```python
from build123d import *

# Parameters (mm, degrees)
F0_W     = 127
F0_H     = 63.5
F0_R     = 19.05
F1_DEPTH = 25.4
F2_W     = 6.35
F2_H     = 63.5
F2_W_2   = 12.7
F3_DEPTH = 2.54
F5_DEPTH = 66.04
F6_R     = 4.7625
F7_DEPTH = 12.7


with BuildPart() as f1:
    # F0 (on Front) → F1 (new body)
    with BuildSketch(Plane.XZ):
        with Locations((1.798787, 0)):
            Rectangle(F0_W, F0_H)
        Circle(F0_R, mode=Mode.SUBTRACT)
    extrude(amount=F1_DEPTH)

    # F2 (on face) → F3 (cut)
    with BuildSketch(Plane.XZ.offset(25.4)):
        with Locations((-55.986213, 0)):
            Rectangle(F2_W, F2_H)
        Rectangle(F2_W_2, F2_H)
    extrude(amount=-F3_DEPTH, mode=Mode.SUBTRACT)

    # F4 (on face) → F5 (cut)
    with BuildSketch(Plane(origin=(0, 0, -31.75), x_dir=(1, 0, 0), z_dir=(0, 0, -1))):
        Polygon((44.45, 25.4), (31.75, 25.4), (28.817061, 20.32), (47.382939, 20.32), align=None)
    extrude(amount=-F5_DEPTH, mode=Mode.SUBTRACT)

    # F6 (on face) → F7 (join)
    with BuildSketch(Plane.YZ.offset(65.298787)):
        with Locations((-12.7, 0)):
            Circle(F6_R)
    extrude(amount=F7_DEPTH)


solid = f1.part
```
Geometry: final body of the model. Coordinates: model frame, mm. A direction names the side the tool comes from. Give positions to 0.01 mm unless a question says otherwise; leave off trailing zeros. Loops run counter-clockwise (first coordinate to the right, second up) from the corner with the lowest first, then second, coordinate; pieces in that order, holes last. Notation, with made-up numbers: (55.5, 7) - (75.5, 7) arc R22 cw to (75.5, 20) - close; hole circle Ø11 at (86.5, 83.5). An arc over 180 degrees is marked (long way). Answer as CSV lines item,"result". Start each with the question number.
(1) Mould query, pull axis X, two halves, no side actions, for faces 1 (the face through (-30, -25.4, 0)), 2 (the face through (-61.701, -13, 0)), 3 (the face through (-6.35, -24, -25)), 4 (the face through (65.299, -18, 0)). Classes: +X half, -X half, draft (parallel to the pull), parting line (faces both ways), or undercut.
(2) Section query B-B (z = 0). Output: boundary loops of the cut face in (x, y).
(3) Section query A-A (y = -12.7). Output: boundary loops of the cut face in (x, z), and give its area (3 significant figures).
(4) Reachability of faces 5 (the face through (18.17, -12.52, 5.72)), 6 (the face through (30.304, -22.896, -0.444)), 7 (the face through (71.56, -8.3, -1.82)), 8 (the face through (6.35, -24, -25)) from +Z, -Z, +X, -X, +Y, -Y: full face, straight path, thin tool, end or side. Return the list, or none.
(5) Section query D-D (z = -25.5). Output: boundary loops of the cut face in (x, y), and give its area (3 significant figures).
(6) Ray query, line 1 along Z through (x, y) = (0, -9.5); line 2 along X through (y, z) = (-11.75, 0); line 3 along X through (y, z) = (-7.5, 0). Return the intervals inside material, ascending. Write a range as [from, to].
(7) Section query C-C (x = 0). Output: boundary loops of the cut face in (y, z), and give its area (3 significant figures).
(8) Pin query (flat end, axial travel): P1, Ø2, axis at y = -15, z = 21, coming from the +X side; P2, Ø9.5, axis at x = 38, z = 6, coming from the -Y side; P3, Ø10, axis at x = -1, z = 28.5, coming from the -Y side. Return the tip coordinate at first contact, or that it passes through.
Worked answers:
1,face 1,"draft"
1,face 2,"-X half"
1,face 3,"undercut"
1,face 4,"+X half"
2,outline,"(-61.7, -25.4) - (-59.16, -25.4) - (-59.16, -22.86) - (-52.81, -22.86) - (-52.81, -25.4) - (-19.05, -25.4) - (-19.05, 0) - (-61.7, 0) - close; (19.05, -25.4) - (31.75, -25.4) - (28.82, -20.32) - (47.38, -20.32) - (44.45, -25.4) - (65.3, -25.4) - (65.3, -17.46) - (78, -17.46) - (78, -7.94) - (65.3, -7.94) - (65.3, 0) - (19.05, 0) - close"
3,outline,"(-61.7, -31.75) - (65.3, -31.75) - (65.3, -4.76) - (78, -4.76) - (78, 4.76) - (65.3, 4.76) - (65.3, 31.75) - (-61.7, 31.75) - close; hole circle Ø38.1 at (0, 0)"
3,area,"7,050 mm^2"
4,face 5,"+Y, -Y"
4,face 6,"+Z, -Z"
4,face 7,"+X"
4,face 8,"+Z, -Z, -Y"
5,outline,"(-61.7, -25.4) - (-59.16, -25.4) - (-59.16, -22.86) - (-52.81, -22.86) - (-52.81, -25.4) - (-6.35, -25.4) - (-6.35, -22.86) - (6.35, -22.86) - (6.35, -25.4) - (31.75, -25.4) - (28.82, -20.32) - (47.38, -20.32) - (44.45, -25.4) - (65.3, -25.4) - (65.3, 0) - (-61.7, 0) - close"
5,area,"3,100 mm^2"
6,line 1,"z = [-31.75, -19.05], [19.05, 31.75]"
6,line 2,"x = [-61.7, -19.05], [19.05, 78]"
6,line 3,"x = [-61.7, -19.05], [19.05, 65.3]"
7,outline,"(-22.86, -31.75) - (0, -31.75) - (0, -19.05) - (-22.86, -19.05) - close; (-22.86, 19.05) - (0, 19.05) - (0, 31.75) - (-22.86, 31.75) - close"
7,area,"581 mm^2"
8,P1,"stops at x = 65.3"
8,P2,"stops at y = -20.32"
8,P3,"stops at y = -22.86"
